```python
from build123d import *

# Parameters (mm, degrees)
F2_DEPTH  = 81
F3_DEPTH  = 10
F4_START  = -71
F4_DEPTH  = 10
F8_R      = 15
F9_DEPTH  = 1.6
F10_W     = 15.4
F10_H     = 14.6
F11_DEPTH = 1.6
F12_W     = 18
F12_H     = 18
F13_DEPTH = 1.6


# Not quite as in the source:
# - a feature names something its author has since deleted; it is built from what else it names


with BuildPart() as f2:
    # F1 (on offset) → F2 (new body)
    with BuildSketch(Plane.XZ.offset(40.5)):
        Polygon((76.55, 0), (76.55, 1.6), (-76.55, 1.6), (-76.55, 0), (-70.55, 0), (-68.15, 0), (-62.15, 0), (-37.15, 0), (-31.15, 0), (-28.75, 0), (-22.75, 0), (22.75, 0), (28.75, 0), (31.15, 0), (37.15, 0), (62.15, 0), (68.15, 0), (70.55, 0), align=None)
    extrude(amount=-F2_DEPTH)

    # F1 (on offset) → F3 (join)
    with BuildSketch(Plane.XZ.offset(40.5)):
        Polygon((-62.15, 0), (-68.15, 0), (-68.15, -6), align=None)
        Polygon((-31.15, 0), (-37.15, 0), (-31.15, -6), align=None)
        Polygon((-22.75, 0), (-28.75, 0), (-28.75, -6), align=None)
        Polygon((-70.55, 0), (-76.55, 0), (-70.55, -6), align=None)
    extrude(amount=-F3_DEPTH)

    # F1 (on offset) → F4 (join)
    with BuildSketch(Plane.XZ.offset(40.5).offset(F4_START)):
        Polygon((-62.15, 0), (-68.15, 0), (-68.15, -6), align=None)
        Polygon((-31.15, 0), (-37.15, 0), (-31.15, -6), align=None)
        Polygon((-22.75, 0), (-28.75, 0), (-28.75, -6), align=None)
        Polygon((-70.55, 0), (-76.55, 0), (-70.55, -6), align=None)
    extrude(amount=-F4_DEPTH)

    # F7: F2 across plane


with BuildPart() as f2_1:
    add(f2.part)
    add(f2.part.mirror(Plane.YZ))

    # F8 (on face) → F9 (cut)
    with BuildSketch(Plane.XY.offset(1.6)):
        with Locations((0, -15.5)):
            Circle(F8_R)
    extrude(amount=-F9_DEPTH, mode=Mode.SUBTRACT)

    # F10 (on face) → F11 (cut)
    with BuildSketch(Plane.XY.offset(1.6)):
        with Locations((-49.65, 20.6)):
            Rectangle(F10_W, F10_H)
        with Locations((49.65, 20.6)):
            Rectangle(F10_W, F10_H)
    extrude(amount=-F11_DEPTH, mode=Mode.SUBTRACT)

    # F12 (on Top) → F13 (cut)
    with BuildSketch(Plane.XY):
        with Locations((-49.65, -15.7)):
            Rectangle(F12_W, F12_H)
        with Locations((49.65, -15.7)):
            Rectangle(F12_W, F12_H)
    extrude(amount=F13_DEPTH, mode=Mode.SUBTRACT)


solid = f2_1.part
```
Source: CAD feature listing. Evaluate the final solid. Frame: model axes, mm. A direction names the side the tool comes from. Coordinates: 2 decimals unless noted, no trailing zeros. Order: outer loops, then holes, each group sorted by start corner. A loop starts at its lowest first (then second) coordinate and runs counter-clockwise, first axis right, second up. Notation, with made-up numbers: (15.25, 56) - (34.25, 56) arc R23 cw to (34.25, 77) - close; hole circle Ø10 at (84, 22). An arc over 180 degrees is marked (long way). One line per item, written item: value.
1) Cut plane C-C on y = 23. Output: boundary loops of the cut face in (x, z), plus the area to 3 significant figures.
Computed values:
outline: (-76.55, 0) - (-57.35, 0) - (-57.35, 1.6) - (-76.55, 1.6) - close; (-41.95, 0) - (41.95, 0) - (41.95, 1.6) - (-41.95, 1.6) - close; (57.35, 0) - (76.55, 0) - (76.55, 1.6) - (57.35, 1.6) - close
area: 196 mm^2
2) Reachability of faces 1 (the face through (72, 30.5, -2)), 2 (the face through (73.59, -35.57, -2.96)), 3 (the face through (-31.15, -36, -3)) from +Z, -Z, +X, -X, +Y, -Y: full face, straight path, thin tool, end or side. Return the list, or none.
Computed values:
face 1: -Z, +X, -X
face 2: -Z, +X, +Y, -Y
face 3: -Z, +Y, -Y
3) Contact query for a flat-ended pin moving along its axis: pin 1 (4 mm diameter, centred on y = 29.5, z = -4.5, fed in from -X). Output: stop coordinate, or through.
Computed values:
pin 1: stops at x = -73.78
4) Cut plane A-A on y = -15.5. Output: boundary loops of the cut face in (x, z), plus the area to 3 significant figures.
Computed values:
outline: (-76.55, 0) - (-58.65, 0) - (-58.65, 1.6) - (-76.55, 1.6) - close; (-40.65, 0) - (-15, 0) - (-15, 1.6) - (-40.65, 1.6) - close; (15, 0) - (40.65, 0) - (40.65, 1.6) - (15, 1.6) - close; (58.65, 0) - (76.55, 0) - (76.55, 1.6) - (58.65, 1.6) - close
area: 139 mm^2
5) Cut plane D-D on x = 54. Output: boundary loops of the cut face in (y, z), plus the area to 3 significant figures.
Computed values:
outline: (-40.5, 0) - (-24.7, 0) - (-24.7, 1.6) - (-40.5, 1.6) - close; (-6.7, 0) - (13.3, 0) - (13.3, 1.6) - (-6.7, 1.6) - close; (27.9, 0) - (40.5, 0) - (40.5, 1.6) - (27.9, 1.6) - close
area: 77.4 mm^2
6) Cut plane B-B on x = 12. Output: boundary loops of the cut face in (y, z).
Computed values:
outline: (-40.5, 0) - (-24.5, 0) - (-24.5, 1.6) - (-40.5, 1.6) - close; (-6.5, 0) - (40.5, 0) - (40.5, 1.6) - (-6.5, 1.6) - close
7) Ray query, line 1 (X direction, y = 19.5, z = 1); line 2 (Y direction, x = 26, z = -2.5); line 3 (Z direction, x = -68.5, y = 3). Return the intervals inside material, ascending. Write a range as [from, to].
Computed values:
line 1: x = [-76.55, -57.35], [-41.95, 41.95], [57.35, 76.55]
line 2: y = [-40.5, -30.5], [30.5, 40.5]
line 3: z = [0, 1.6]
